```python
from build123d import *

# Parameters (mm, degrees)
F1_R     = 51.165041
F2_DEPTH = 50.8
F0_W     = 101.995886
F0_H     = 85.735648
F3_DEPTH = 25.4


with BuildPart() as f2:
    # F1 (on face) → F2 (new body)
    with BuildSketch(Plane.XY):
        with Locations((0, 45.085132)):
            Circle(F1_R)
    extrude(amount=F2_DEPTH)

    # F0 (on Top) → F3 (join)
    with BuildSketch(Plane.XY):
        Rectangle(F0_W, F0_H)
    extrude(amount=-F3_DEPTH)


solid = f2.part
```
Geometry check sheet. Reference: the model listing, model coordinates, mm. A direction names the side the tool comes from. Coordinates: 2 decimals unless noted, no trailing zeros. Order: outer loops, then holes, each group sorted by start corner. A loop starts at its lowest first (then second) coordinate and runs counter-clockwise, first axis right, second up. Notation, with made-up numbers: M 2.5,-6.75 L 53.5,-6.75 A25 cw 53.5,14.25 Z; hole C 24,-34.75 d5. An arc over 180 degrees is marked long. One line per question, with ' | ' between items. Start each with the question number.
Item 1: Material ranges on L1, parallel to Z at x = -11, y = -24; L2, parallel to Z at x = -15, y = 49; L3, parallel to X at y = 24, z = -6, recorded low to high. Write a range as [from, to].
Item 2: Set-up check for faces 1 (the cylindrical face through (48.802, 60.454, 25.044)), 2 (the flat face through (-1, 42.868, -13)), 3 (the flat face through (-1, 46, 50.8)): record each of +Z, -Z, +X, -X, +Y, -Y from which the full face is reachable in a straight line by a thin tool's end or side.
Item 3: Cross-section at A-A on x = 0. Enter the section's corners in (y, z), then the cut area to 3 significant figures.
Item 4: Cross-section at B-B on y = 3. Enter the section's corners in (x, z), then the cut area to 3 significant figures.
Item 5: Cross-section at D-D on y = 52.5. Enter the section's corners in (x, z).
Item 6: Gauge pin test, flat ends, axial feed: pin 1 (12 mm diameter, centred on y = 27, z = -16, fed in from -X); pin 2 (12 mm diameter, centred on y = 9, z = 11.5, fed in from -X); pin 3 (7.5 mm diameter, centred on x = 22.5, z = -14.5, fed in from +Y). Record the tip position at first contact, or that the pin passes through.
Item 7: Cross-section at C-C on z = -19. Enter the section's corners in (x, y), then the cut area to 3 significant figures.
Findings:
1) L1: z = [-25.4, 0] | L2: z = [0, 50.8] | L3: x = [-51, 51]
2) face 1: +Z | face 2: -Z, +X, -X, +Y | face 3: +Z, +X, -X, +Y, -Y
3) outline: M -42.87,-25.4 L 42.87,-25.4 L 42.87,0 L 96.25,0 L 96.25,50.8 L -6.08,50.8 L -6.08,0 L -42.87,0 Z | area: 7,380 mm²
4) outline: M -51,-25.4 L 51,-25.4 L 51,0 L 29.1,0 L 29.1,50.8 L -29.1,50.8 L -29.1,0 L -51,0 Z | area: 5,550 mm²
5) outline: M -50.62,0 L 50.62,0 L 50.62,50.8 L -50.62,50.8 Z
6) pin 1: stops at x = -51 | pin 2: stops at x = -41.39 | pin 3: stops at y = 42.87
7) outline: M -51,-42.87 L 51,-42.87 L 51,42.87 L -51,42.87 Z | area: 8,740 mm²
